Could you check a few things on this model? Use its own coordinates, in mm. A direction names the side the tool comes from. Give positions to 0.01 mm unless a question says otherwise; leave off trailing zeros. Loops run counter-clockwise (first coordinate to the right, second up) from the corner with the lowest first, then second, coordinate; pieces in that order, holes last. Notation, with made-up numbers: (19.5, -16) -> (51.5, -16) arc R22 ccw to (51.5, 20) -> close; hole circle Ø5 at (4.25, 59). An arc over 180 degrees is marked (long way). Put each result on its own line as item: value.
```python
from build123d import *

# Parameters (mm, degrees)
F0_W     = 33
F0_H     = 34
F1_DEPTH = 6
F3_W     = 6
F3_H     = 15
F4_DEPTH = 6
F2_R     = 1.6
F5_DEPTH = 6


with BuildPart() as f1:
    # F0 (on Top) → F1 (new body)
    with BuildSketch(Plane.XY):
        Rectangle(F0_W, F0_H)
    extrude(amount=F1_DEPTH)

    # F3 (on Top) → F4 (join)
    with BuildSketch(Plane.XY):
        with Locations((-19.5, 0)):
            Rectangle(F3_W, F3_H)
        with Locations((19.5, 0)):
            Rectangle(F3_W, F3_H)
    extrude(amount=F4_DEPTH)

    # F2 (on face) → F5 (cut, through all)
    with BuildSketch(Plane.XY.offset(6)):
        with Locations((-10, -11.85)):
            Circle(F2_R)
        with Locations((10, -11.85)):
            Circle(F2_R)
        with Locations((0, 11.85)):
            Circle(F2_R)
    extrude(amount=-F5_DEPTH, mode=Mode.SUBTRACT)


solid = f1.part
```
1. I need wall thicknesses on line 1 (X direction, y = -12, z = 3.05); line 2 (Y direction, x = 0, z = 4.55); line 3 (X direction, y = 15, z = 2.75). Which ranges of each line are inside material? Lowest first, please.
Recorded:
line 1: x = -16.5 to -11.59, -8.41 to 8.41, 11.59 to 16.5
line 2: y = -17 to 10.25, 13.45 to 17
line 3: x = -16.5 to 16.5
2. Thinking about a two-plate mould opening in Y: for faces 1 (the face through (-22.5, 0, 3)), 2 (the face through (-0.35, 10.29, 3.04)), 3 (the face through (-20, -7.5, 3)), 4 (the face through (-11.27, -12.82, 3.04)), which applies, pulls with the +Y half, pulls with the -Y half, needs draft (parallel to the pull), parting line crosses it, or undercut?
Recorded:
face 1: needs draft
face 2: undercut
face 3: pulls with the -Y half
face 4: undercut
3. If we section it at A-A (x = 10): List the corners of the cut face in (y, z) for me.
Recorded:
outline: (-17, 0) -> (-13.45, 0) -> (-13.45, 6) -> (-17, 6) -> close; (-10.25, 0) -> (17, 0) -> (17, 6) -> (-10.25, 6) -> close
4. If we section it at B-B (y = -11.85): List the corners of the cut face in (x, z) for me, then the cut area to 3 significant figures.
Recorded:
outline: (-16.5, 0) -> (-11.6, 0) -> (-11.6, 6) -> (-16.5, 6) -> close; (-8.4, 0) -> (8.4, 0) -> (8.4, 6) -> (-8.4, 6) -> close; (11.6, 0) -> (16.5, 0) -> (16.5, 6) -> (11.6, 6) -> close
area: 160 mm^2
5. If we section it at D-D (y = 11.85): List the corners of the cut face in (x, z) for me, then the cut area to 3 significant figures.
Recorded:
outline: (-16.5, 0) -> (-1.6, 0) -> (-1.6, 6) -> (-16.5, 6) -> close; (1.6, 0) -> (16.5, 0) -> (16.5, 6) -> (1.6, 6) -> close
area: 179 mm^2
6. For faces 5 (the face through (16.5, -12, 3)), 6 (the face through (19, 7.5, 3)), 7 (the face through (-16.5, 12, 3)), which set-ups out of +Z, -Z, +X, -X, +Y, -Y let a thin tool reach every point of the face, with its end or its side?
Recorded:
face 5: +Z, -Z, +X, -Y
face 6: +Z, -Z, +X, +Y
face 7: +Z, -Z, -X, +Y
7. I'm going to push flat-ended pins straight in: pin 1 (1.9 mm diameter, centred on x = -10, y = -11.85, fed in from +Z); pin 2 (3 mm diameter, centred on y = 12.5, z = 4, fed in from -X); pin 3 (1.8 mm diameter, centred on x = -18.5, z = 3, fed in from -Y); pin 4 (3 mm diameter, centred on y = -13, z = 2.5, fed in from +X). Where does each tip first touch, or does it pass through?
Recorded:
pin 1: passes through
pin 2: stops at x = -16.5
pin 3: stops at y = -7.5
pin 4: stops at x = 16.5
8. If we section it at C-C (z = 4.35): List the corners of the cut face in (x, y) for me, then the cut area to 3 significant figures.
Recorded:
outline: (-22.5, -7.5) -> (-16.5, -7.5) -> (-16.5, -17) -> (16.5, -17) -> (16.5, -7.5) -> (22.5, -7.5) -> (22.5, 7.5) -> (16.5, 7.5) -> (16.5, 17) -> (-16.5, 17) -> (-16.5, 7.5) -> (-22.5, 7.5) -> close; hole circle Ø3.2 at (-10, -11.85); hole circle Ø3.2 at (0, 11.85); hole circle Ø3.2 at (10, -11.85)
area: 1,280 mm^2
